```python
from build123d import *

# Parameters (mm, degrees)
SKETCH1_W           = 45
SKETCH1_H           = 20.7
SKETCH1_R           = 1.5
BOSS_EXTRUDE1_DEPTH = 6
SKETCH3_W           = 18
SKETCH3_H           = 5
CUT_EXTRUDE1_DEPTH  = 3


with BuildPart() as part:
    # Sketch1 → Boss-Extrude1 (new body)
    with BuildSketch(Plane.XY):
        with Locations((4.046614158, 1.856007179)):
            Rectangle(SKETCH1_W, SKETCH1_H)
        with Locations((16.546614158, 8.506007179)):
            Circle(SKETCH1_R, mode=Mode.SUBTRACT)
        with Locations((-8.453385842, 8.506007179)):
            Circle(SKETCH1_R, mode=Mode.SUBTRACT)
    extrude(amount=BOSS_EXTRUDE1_DEPTH)

    # Sketch3 → Cut-Extrude1 (cut)
    with BuildSketch(Plane.XY.offset(6)):
        with Locations((4.046614158, 9.706007179)):
            Rectangle(SKETCH3_W, SKETCH3_H)
    extrude(amount=-CUT_EXTRUDE1_DEPTH, mode=Mode.SUBTRACT)


solid = part.part
```
Design review of the part built by this model. Coordinates are the model's own, in mm. A direction names the side the tool comes from. Round coordinates to 2 decimals unless told otherwise and drop trailing zeros. Write each loop counter-clockwise with the first axis right and the second up, starting at its lowest first coordinate (ties: lowest second). Pieces come first, ordered by that corner, then holes.
Item 1: Clearance check with flat-ended pins moving along their axes: pin 1 Ø0.9 at (x, z) = (6.5, 4) entering from +Y; pin 2 Ø5.5 at (x, y) = (5.5, 10) entering from +Z. State where each tip first meets the part, or that it passes through.
Item 2: The part is to be moulded in two halves that separate along X. For faces 1 (the flat face through (-4.953, 10, 5)), 2 (the flat face through (26.547, 2, 3)), 3 (the flat face through (4, 7.206, 5)), 4 (the flat face through (4, -8.494, 3)), say which applies: +X half, -X half, draft (parallel to the pull), parting line (faces both ways), or undercut.
Item 3: For probe 1 along X at (y, z) = (11.25, 5.4); probe 2 along Y at (x, z) = (15.5, 1.7); probe 3 along Y at (x, z) = (11.5, 5.65), list the stretches that pass through material, from the lowest coordinate up.
Item 4: We need section B-B on y = 9. Write out the cut boundary in (x, z).
Item 5: We need section A-A on x = -3. Write out the cut boundary in (y, z).
Item 6: For faces 5 (the flat face through (4, 12.206, 2)), 6 (the flat face through (4, 10, 3)), list the 3-axis set-ups (+Z, -Z, +X, -X, +Y, -Y) from which the entire face can be reached by the end or side of a thin tool; tool diameter is ignored.
Item 7: We need section D-D on z = 0.65. Write out the cut boundary in (x, y).
Item 8: We need section C-C on z = 5.15. Write out the cut boundary in (x, y).
Returned:
1. pin 1: stops at y = 7.21
1. pin 2: stops at z = 3
2. face 1: undercut
2. face 2: +X half
2. face 3: undercut
2. face 4: draft
3. probe 1: x = -18.45 to -4.95, 13.05 to 26.55
3. probe 2: y = -8.49 to 7.43, 9.58 to 12.21
3. probe 3: y = -8.49 to 7.21
4. outline: (-18.45, 0) - (-9.87, 0) - (-9.87, 6) - (-18.45, 6) - close; (-7.04, 0) - (15.13, 0) - (15.13, 6) - (13.05, 6) - (13.05, 3) - (-4.95, 3) - (-4.95, 6) - (-7.04, 6) - close; (17.96, 0) - (26.55, 0) - (26.55, 6) - (17.96, 6) - close
5. outline: (-8.49, 0) - (12.21, 0) - (12.21, 3) - (7.21, 3) - (7.21, 6) - (-8.49, 6) - close
6. face 5: +Z, -Z, +X, -X, +Y
6. face 6: +Z, +Y
7. outline: (-18.45, -8.49) - (26.55, -8.49) - (26.55, 12.21) - (-18.45, 12.21) - close; hole circle Ø3 at (-8.45, 8.51); hole circle Ø3 at (16.55, 8.51)
8. outline: (-18.45, -8.49) - (26.55, -8.49) - (26.55, 12.21) - (13.05, 12.21) - (13.05, 7.21) - (-4.95, 7.21) - (-4.95, 12.21) - (-18.45, 12.21) - close; hole circle Ø3 at (-8.45, 8.51); hole circle Ø3 at (16.55, 8.51)
